Source: CAD feature listing. Evaluate the final solid. Frame: model axes, mm. Give positions to 0.01 mm unless a question says otherwise; leave off trailing zeros. Order: outer loops, then holes, each group sorted by start corner. A loop starts at its lowest first (then second) coordinate and runs counter-clockwise, first axis right, second up. Notation, with made-up numbers: M 73,22 L 78,22 A13 cw 78,37 Z; hole C -31,0 d11. An arc over 180 degrees is marked long. Answer in a Markdown table with one row per item. Add a question column.
(1) Section query C-C, the plane x = 5. Return loops of the section in (y, z) (3 decimals), plus the area to 3 significant figures.
(2) Section query A-A, the plane z = 0. Return loops of the section in (x, y) (3 decimals).
(3) Pin query (flat end, axial travel): P1, Ø10, axis at y = 15.5, z = -9.5, coming from the -X side; P2, Ø6, axis at x = 16, y = -1.5, coming from the -Z side; P3, Ø6, axis at x = 7.5, z = 9.5, coming from the +Y side. Return the tip coordinate at first contact, or that it passes through.
(4) Material intervals for line 1 along Z through (x, y) = (11.25, 0) (3 decimals); line 2 along Z through (x, y) = (4.25, 0) (3 decimals); line 3 along X through (y, z) = (15, -13), sorted ascending.
(5) Section query D-D, the plane y = 11.5. Return loops of the section in (x, z).
(6) Mould query, pull axis Z, two halves, no side actions, for faces 1 (the face through (10, 0, -6)), 2 (the face through (8.87, -0.59, -1.13)), 3 (the face through (4.9, -0.7, -3.3)). Classes: pulls with the +Z half, pulls with the -Z half, needs draft (parallel to the pull), parting line crosses it, or undercut.
from build123d import *

# Parameters (mm, degrees)
F0_R     = 3.375
F1_DEPTH = 10
F2_R     = 27.5
F2_R_2   = 3.375
F3_DEPTH = 8
F4_R     = 1.275
F5_DEPTH = 25.4


with BuildPart() as f1:
    # F0 (on Right) → F1 (new body)
    with BuildSketch(Plane.YZ):
        Circle(F0_R)
    extrude(amount=F1_DEPTH)

    # F2 (on face) → F3 (join)
    with BuildSketch(Plane.YZ.offset(10)):
        Circle(F2_R)
        Circle(F2_R_2, mode=Mode.SUBTRACT)
        Circle(F2_R_2)
    extrude(amount=F3_DEPTH)

    # F4 (on face) → F5 (cut)
    with BuildSketch(Plane(origin=(0, 0, 0), x_dir=(0, -1, 0), z_dir=(-1, 0, 0))):
        Circle(F4_R)
    extrude(amount=-F5_DEPTH, mode=Mode.SUBTRACT)


solid = f1.part
Values follow:
| question | item | result |
|---|---|---|
| 1 | outline | C 0,0 d6.75; hole C 0,0 d2.55 |
| 1 | area | 30.7 mm² |
| 2 | outline | M 0,-3.375 L 10,-3.375 L 10,-27.5 L 18,-27.5 L 18,-1.275 L 0,-1.275 Z; M 0,1.275 L 18,1.275 L 18,27.5 L 10,27.5 L 10,3.375 L 0,3.375 Z |
| 3 | P1 | stops at x = 10 |
| 3 | P2 | stops at z = -27.5 |
| 3 | P3 | stops at y = 26.36 |
| 4 | line 1 | z = -27.5 to -1.275, 1.275 to 27.5 |
| 4 | line 2 | z = -3.375 to -1.275, 1.275 to 3.375 |
| 4 | line 3 | x = 10 to 18 |
| 5 | outline | M 10,-24.98 L 18,-24.98 L 18,24.98 L 10,24.98 Z |
| 6 | face 1 | needs draft |
| 6 | face 2 | undercut |
| 6 | face 3 | parting line crosses it |
